Source: CAD feature listing. Evaluate the final solid. Frame: model axes, mm. A direction names the side the tool comes from. Round coordinates to 2 decimals unless told otherwise and drop trailing zeros. Write each loop counter-clockwise with the first axis right and the second up, starting at its lowest first coordinate (ties: lowest second). Pieces come first, ordered by that corner, then holes. Notation, with made-up numbers: M -1.75,8.25 L 7.25,8.25 A33 cw 7.25,45.25 Z; hole C -30,77 d8. An arc over 180 degrees is marked long. Answer in a Markdown table with one row per item. Add a question column.
Item 1: Cut plane A-A on x = 5. Return loops of the section in (y, z), and give its area (3 significant figures).
Item 2: Material intervals for probe 1 along Y at (x, z) = (25, 1.2); probe 2 along X at (y, z) = (7.75, 0.5); probe 3 along Y at (x, z) = (15, 2.3), sorted ascending.
Item 3: Cut plane B-B on z = 0.6. Return loops of the section in (x, y), and give its area (3 significant figures).
Item 4: Cut plane D-D on y = 2.5. Return loops of the section in (x, z).
Item 5: Contact query for a flat-ended pin moving along its axis: pin 1 (2.5 mm diameter, centred on x = 5, y = 7.5, fed in from +Z). Output: stop coordinate, or through.
Item 6: Mould query, pull axis Y, two halves, no side actions, for faces 1 (the face through (15, 11, 0)), 2 (the face through (0.6, 14.43, 1.48)), 3 (the face through (3.35, 7.57, 1.52)). Classes: released by +Y, released by -Y, zero draft, split by the parting line, or undercut.
Item 7: Set-up query: faces 4 (the face through (8.506, 7.786, 2.26)), 5 (the face through (0, 8, 1)). Return all of +Z, -Z, +X, -X, +Y, -Y with unobstructed straight access to the full face (end or side cutting, diameter ignored); none if empty.
Item 8: Cut plane C-C on y = 6.25. Return loops of the section in (x, z).
from build123d import *

# Parameters (mm, degrees)
EXTRUDE_1_DEPTH     = 3
SKETCH_2_R          = 6.5
CUT_EXTRUDE_1_DEPTH = 1.5
SKETCH_3_R          = 3.25
CUT_EXTRUDE_2_DEPTH = 34.674916481
SKETCH_4_R          = 1.65
CUT_EXTRUDE_3_DEPTH = 34.674916481


with BuildPart() as part:
    # Эскиз1 → Бобышка-Вытянуть1 (new body)
    with BuildSketch(Plane.XY):
        with BuildLine():
            Line((2, 0), (28, 0))
            ThreePointArc((28, 0), (29.414213562, 0.585786438), (30, 2))
            Line((30, 2), (30, 13))
            ThreePointArc((30, 13), (29.414213562, 14.414213562), (28, 15))
            Line((28, 15), (2, 15))
            ThreePointArc((2, 15), (0.585786438, 14.414213562), (0, 13))
            Line((0, 13), (0, 2))
            ThreePointArc((0, 2), (0.585786438, 0.585786438), (2, 0))
        make_face()
    extrude(amount=EXTRUDE_1_DEPTH)

    # Эскиз2 → Вырез-Вытянуть1 (cut)
    with BuildSketch(Plane.XY.offset(3)):
        with Locations((15, 7.5)):
            Circle(SKETCH_2_R)
    extrude(amount=-CUT_EXTRUDE_1_DEPTH, mode=Mode.SUBTRACT)

    # Эскиз3 → Вырез-Вытянуть2 (cut, through all)
    with BuildSketch(Plane.XY.offset(3)):
        with Locations((15, 7.5)):
            Circle(SKETCH_3_R)
    extrude(amount=-CUT_EXTRUDE_2_DEPTH, mode=Mode.SUBTRACT)

    # Эскиз4 → Вырез-Вытянуть3 (cut, through all)
    with BuildSketch(Plane.XY.offset(3)):
        with Locations((5, 7.5)):
            Circle(SKETCH_4_R)
        with Locations((25, 7.5)):
            Circle(SKETCH_4_R)
    extrude(amount=-CUT_EXTRUDE_3_DEPTH, mode=Mode.SUBTRACT)


solid = part.part
Results below:
| question | item | result |
|---|---|---|
| 1 | outline | M 0,0 L 5.85,0 L 5.85,3 L 0,3 Z; M 9.15,0 L 15,0 L 15,3 L 9.15,3 Z |
| 1 | area | 35.1 mm2 |
| 2 | probe 1 | 0 to 5.85, 9.15 to 15 |
| 2 | probe 2 | 0 to 3.37, 6.63 to 11.76, 18.24 to 23.37, 26.63 to 30 |
| 2 | probe 3 | 0 to 1, 14 to 15 |
| 3 | outline | M 0,2 A2 ccw 2,0 L 28,0 A2 ccw 30,2 L 30,13 A2 ccw 28,15 L 2,15 A2 ccw 0,13 Z; hole C 5,7.5 d3.3; hole C 15,7.5 d6.5; hole C 25,7.5 d3.3 |
| 3 | area | 396 mm2 |
| 4 | outline | M 0,0 L 30,0 L 30,3 L 19.15,3 L 19.15,1.5 L 10.85,1.5 L 10.85,3 L 0,3 Z |
| 5 | pin 1 | through |
| 6 | face 1 | zero draft |
| 6 | face 2 | released by +Y |
| 6 | face 3 | undercut |
| 7 | face 4 | +Z |
| 7 | face 5 | +Z, -Z, -X, +Y, -Y |
| 8 | outline | M 0,0 L 3.92,0 L 3.92,3 L 0,3 Z; M 6.08,0 L 12,0 L 12,1.5 L 8.62,1.5 L 8.62,3 L 6.08,3 Z; M 18,0 L 23.92,0 L 23.92,3 L 21.38,3 L 21.38,1.5 L 18,1.5 Z; M 26.08,0 L 30,0 L 30,3 L 26.08,3 Z |
